Part model, mm, in its own coordinate system. A direction names the side the tool comes from. Round coordinates to 2 decimals unless told otherwise and drop trailing zeros. Order: outer loops, then holes, each group sorted by start corner. A loop starts at its lowest first (then second) coordinate and runs counter-clockwise, first axis right, second up. Notation, with made-up numbers: M 46.5,61.25 L 60.5,61.25 A29 ccw 60.5,81.25 Z; hole C 26.5,-0.5 d4. An arc over 180 degrees is marked long. One line per question, with ' | ' between items.
Autodesk Inventor part; units mm, degrees
ref_plane "Start plane" through (0, 0, 0) normal (0, 0, 1) x (1, 0, 0)
ref_plane "End plane" through (0, 0, 1295.4) normal (0, 0, 1) x (1, 0, 0)
ref_plane "YZ Plane" through (0, 0, 0) normal (1, 0, 0) x (0, 1, 0)
ref_plane "Start plane" through (0, 0, 0) normal (0, 0, 1) x (1, 0, 0)
ref_plane "End plane" through (0, 0, 1295.4) normal (0, 0, 1) x (1, 0, 0)
sketch "Sketch" plane through (0, 0, 0) normal (0, 0, 1) x (1, 0, 0)
  line L0 (0, 76.2) -> (0, 0)
  line L1 (0, 0) -> (50.8, 0)
  line L2 (50.8, 0) -> (50.8, 2.7625)
  line L3 (48.8, 4.7625) -> (12.6365, 4.7625)
  line L4 (4.7625, 12.6365) -> (4.7625, 74.2)
  line L5 (2.7625, 76.2) -> (0, 76.2)
  line L6 (-7.0414, 0) -> (21.5385, 0) construction
  line L7 (0, -8.0414) -> (0, 34.5385) construction
  arc A0 (4.7625, 12.6365) -> (12.6365, 4.7625) centre (12.6365, 12.6365) ccw
  arc A1 (50.8, 2.7625) -> (48.8, 4.7625) centre (48.8, 2.7625) ccw
  arc A2 (4.7625, 74.2) -> (2.7625, 76.2) centre (2.7625, 74.2) ccw
  line L8 (0, 93.5453) -> (0, -24.9725) construction
  line L9 (-18.6925, 0) -> (62.8653, 0) construction
  point P0 (50.8, 4.7625)
  point P1 (4.7625, 4.7625)
  point P2 (4.7625, 76.2)
  dimension "d12" = 4.7625
  dimension "d13" = 76.2
  dimension "d14" = 50.8
  dimension "d15" = 0
  dimension "d16" = 4.7625
  dimension "d17" = 0
  dimension "d18" = 7.874
  dimension "d19" = 2
extrude "Body" add sketch "Sketch" along normal up to surface (1295.4 mm away) from surface at 0
sketch "Sketch3" plane through (0, 0, 0) normal (0, 0, 1) x (1, 0, 0)
  line L0 (0, 0) -> (10, 0)
ref_plane "Work Plane3" through (0, 0, 0) normal (0, -1, 0) x (1, 0, 0)
sketch "Sketch4" plane through (0, 0, 0) normal (0, -1, 0) x (1, 0, 0)
  line L0 (-2, 0) -> (12, 0)
  line L1 (-2, 1295.4) -> (12, 1295.4)
  dimension "d23" = 1295.4
equation "\"d12\" = G_T"
equation "\"d13\" = G_H"
equation "\"d14\" = G_W"
equation "\"d16\" = G_T"
equation "\"d18\" = G_IR"
equation "\"d4\" = G_L"
equation "\"G_W\" = 50.8"
equation "\"G_H\" = 76.2"
equation "\"G_T\" = 4.7625"
equation "\"G_ER\" = 4.064"
equation "\"G_IR\" = 7.874"
equation "\"G_L\" = d23"
equation "\"ex\" = 0"
equation "\"ey\" = 0"
equation "\"G_OFFSET_START\" = 0"
equation "\"G_OFFSET_END\" = 0"
equation "\"d21\" = G_OFFSET_END + B_L"
equation "\"B_L\" = 1295.4"
properties part number "ANSI L 3 x 2 x 3_16 00000003"
1) Saw through at A-A (z = 947.5). List the corners of the cut face in (x, y).
The answers:
outline: M 0,0 L 50.8,0 L 50.8,2.76 A2 ccw 48.8,4.76 L 12.64,4.76 A7.87 cw 4.76,12.64 L 4.76,74.2 A2 ccw 2.76,76.2 L 0,76.2 Z
2) Which spindle directions (+Z, -Z, +X, -X, +Y, -Y) get a long thin tool onto all of the face, cutting with end or side? Do faces 1 (the face through (31, 4.762, 639)), 2 (the face through (25, 0, 639)). Say none if no direction does.
The answers:
face 1: +Z, -Z, +X, +Y | face 2: +Z, -Z, +X, -X, -Y
3) Probe line 1 (Y direction, x = 19, z = 656.5); line 2 (Y direction, x = 5.5, z = 287). List the from-to ranges inside material, lowest first. Write a range as [from, to].
The answers:
line 1: y = [0, 4.76] | line 2: y = [0, 9.31]
4) Saw through at B-B (y = 24). List the corners of the cut face in (x, z).
The answers:
outline: M 0,0 L 4.76,0 L 4.76,1295.4 L 0,1295.4 Z
5) Drop flat-ended pins along their axis: pin 1 (4 mm diameter, centred on y = 8.5, z = 918, fed in from +X); pin 2 (1 mm diameter, centred on y = 48.5, z = 346.5, fed in from +X); pin 3 (4 mm diameter, centred on x = 35, z = 629.5, fed in from +Y). Give the stop position or say it passes through.
The answers:
pin 1: stops at x = 7.7 | pin 2: stops at x = 4.76 | pin 3: stops at y = 4.76
